Source: CAD feature listing. Evaluate the final solid. Frame: model axes, mm. Face numbers are marked on the shaded views. A direction names the side the tool comes from. Give positions to 0.01 mm unless a question says otherwise; leave off trailing zeros. Loops run counter-clockwise (first coordinate to the right, second up) from the corner with the lowest first, then second, coordinate; pieces in that order, holes last. Notation, with made-up numbers: (57.5, -25.5) - (111.5, -25.5) arc R20 ccw to (111.5, 9.5) - close; hole circle Ø4 at (45, 61.25). An arc over 180 degrees is marked (long way). Write each question's results on one line, items separated by ' | '. Start each with the question number.
(1) Cut plane C-C on y = -30. Return the cut outline in (x, z), then the cut area to 3 significant figures.
(2) Pull-direction query (X, two-part tool) for the marked faces 3, 4 and 5; classes: pulls with the +X half, pulls with the -X half, needs draft (parallel to the pull), parting line crosses it, or undercut.
(3) Material intervals for line 1 along Z through (x, y) = (0, -5.75) (3 decimals); line 2 along Y through (x, z) = (-3, 3); line 3 along Y through (x, z) = (-0.5, -2.5), sorted ascending. Write a range as [from, to].
(4) Contact query for flat-ended pins moving along their axis: pin 1 (1 mm diameter, centred on y = -6.5, z = -3.5, fed in from -X); pin 2 (1.9 mm diameter, centred on x = -1.5, z = 1.5, fed in from +Y); pin 3 (5 mm diameter, centred on x = -3.5, y = -41.5, fed in from +Z). Output: stop coordinate, or through.
(5) Reachability of the marked faces 1 and 2 from +Z, -Z, +X, -X, +Y, -Y: full face, straight path, thin tool, end or side. Return the list, or none.
from build123d import *

# Parameters (mm, degrees)
SKETCH1_R           = 4.95935
BOSS_EXTRUDE1_DEPTH = 1.5875
SKETCH2_R           = 3.81
BOSS_EXTRUDE2_DEPTH = 6.35
SKETCH3_R           = 4.95935
BOSS_EXTRUDE4_DEPTH = 42.8625
CHAMFER1_SIZE       = 0.254
SKETCH4_R           = 3.175
CUT_EXTRUDE1_DEPTH  = 7.9375


with BuildPart() as part:
    # Sketch1 → Boss-Extrude1 (new body)
    with BuildSketch(Plane(origin=(0, 0, 0), x_dir=(1, 0, 0), z_dir=(0, 1, 0))):
        Circle(SKETCH1_R)
    extrude(amount=-BOSS_EXTRUDE1_DEPTH)

    # Sketch2 → Boss-Extrude2 (add)
    with BuildSketch(Plane.XZ.offset(1.5875)):
        Circle(SKETCH2_R)
    extrude(amount=BOSS_EXTRUDE2_DEPTH)

    # Sketch3 → Boss-Extrude4 (add)
    with BuildSketch(Plane.XZ.offset(7.9375)):
        Circle(SKETCH3_R)
    extrude(amount=BOSS_EXTRUDE4_DEPTH)

    # Chamfer1
    chamfer1_edges = [part.edges().sort_by_distance(p)[0] for p in [
        (-4.95935, -50.8, 0),
    ]]
    chamfer(chamfer1_edges, length=CHAMFER1_SIZE)

    # Sketch4 → Cut-Extrude1 (cut)
    with BuildSketch(Plane(origin=(0, 0, 0), x_dir=(1, 0, 0), z_dir=(0, 1, 0))):
        Circle(SKETCH4_R)
    extrude(amount=-CUT_EXTRUDE1_DEPTH, mode=Mode.SUBTRACT)


solid = part.part
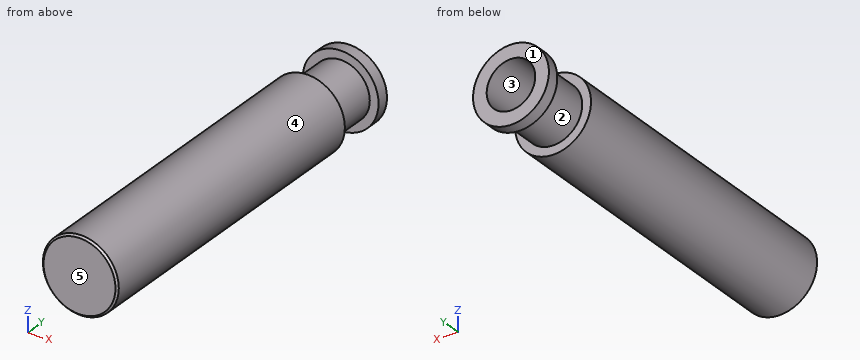
Ans:
1) outline: circle Ø9.92 at (0, 0) | area: 77.3 mm^2
2) face 3: undercut | face 4: parting line crosses it | face 5: needs draft
3) line 1: [-3.81, -3.175], [3.175, 3.81] | line 2: [-50.8, -7.94], [-1.59, 0] | line 3: [-50.8, -7.94]
4) pin 1: x = -2.35 | pin 2: y = -7.94 | pin 3: z = 4.86
5) face 1: +Z, -Z, +X, -X, +Y | face 2: none
